Answer from the drawing. Dimensions are ordinates in mm from the lowest x, y and z of the part. A direction names the side the tool comes from. Round coordinates to 2 decimals unless told otherwise and drop trailing zeros. Loops run counter-clockwise (first coordinate to the right, second up) from the corner with the lowest first, then second, coordinate; pieces in that order, holes last.
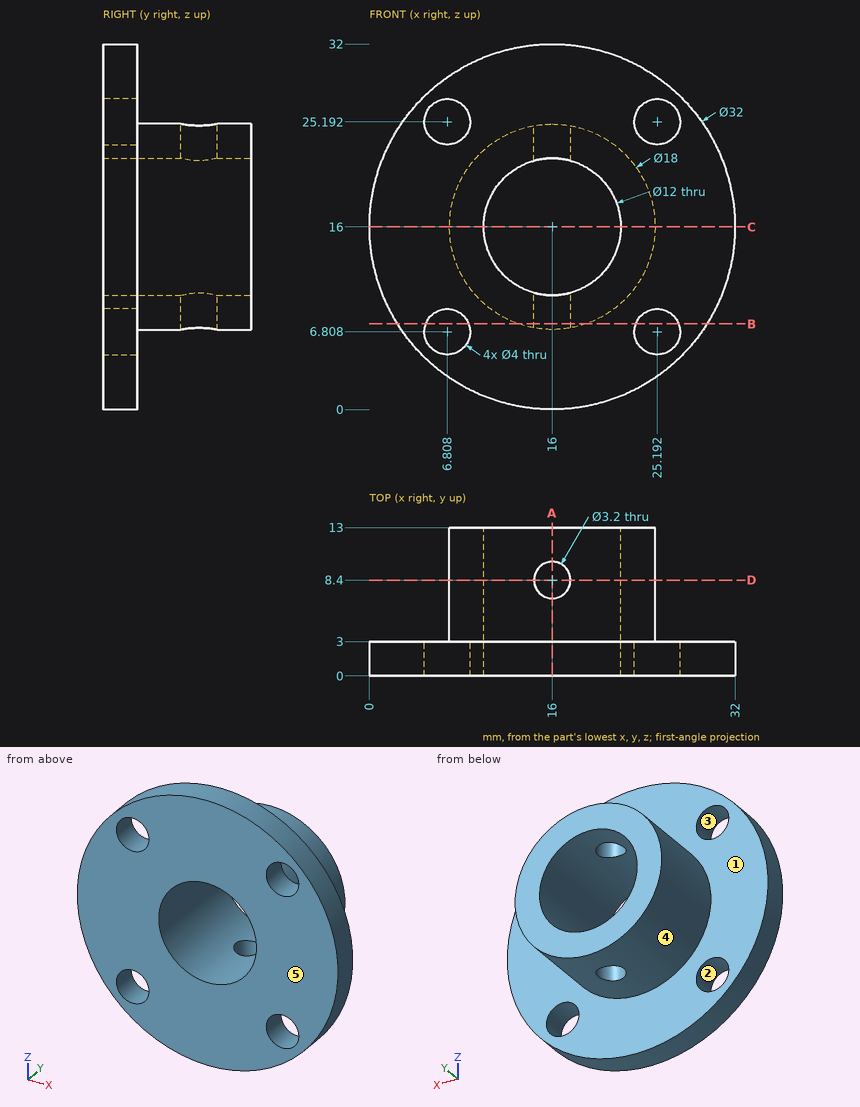
Item 1: Section A-A, the plane x = 16 is taken. Give the vertices of the cut face in (y, z), plus the area to 3 significant figures.
Item 2: Section D-D, the plane y = 8.4 is taken. Give the vertices of the cut face in (x, z), plus the area to 3 significant figures.
Item 3: Section B-B, the plane z = 7.5 is taken. Give the vertices of the cut face in (x, y) (1 decimal), plus the area to 3 significant figures.
Item 4: Determine the mould class of the marked faces 3, 4 and 5 for opening direction X: pulls with the +X half, pulls with the -X half, needs draft (parallel to the pull), parting line crosses it, or undercut.
Item 5: For the marked faces 1 and 2, determine the directions among +Z, -Z, +X, -X, +Y, -Y from which every point of the face is accessible in a straight line to the end or side of a thin tool.
Item 6: Section C-C, the plane z = 16 is taken. Give the vertices of the cut face in (x, y).
Item 7: Straight lines are drawn through the part: line 1 (Y direction, x = 30.5, z = 15); line 2 (Z direction, x = 20.5, y = 11.25) (1 decimal); line 3 (X direction, y = 8.4, z = 9.4). For each, find the intervals that lie inside material, in ascending order.
Item 8: Each of these flat-tipped pins is pushed along its axis until it touches: P1, Ø2, axis at y = 10, z = 9.5, coming from the -X side (1 decimal); P2, Ø1.5, axis at x = 24, y = 10, coming from the +Z side; P3, Ø6, axis at x = 9.5, y = 2.5, coming from the -Z side. Where does it stop, or does it pass through?
Answer below:
1. outline: (0, 0) - (3, 0) - (3, 7) - (6.8, 7) - (6.8, 10) - (0, 10) - close; (0, 22) - (6.8, 22) - (6.8, 25) - (3, 25) - (3, 32) - (0, 32) - close; (10, 7) - (13, 7) - (13, 10) - (10, 10) - close; (10, 22) - (13, 22) - (13, 25) - (10, 25) - close
1. area: 101 mm2
2. outline: (14.4, 7.14) - (14.4, 10.22) arc R6 cw to (14.4, 21.78) - (14.4, 24.86) arc R9 ccw to start; (17.6, 7.14) arc R9 ccw to (17.6, 24.86) - (17.6, 21.78) arc R6 cw to (17.6, 10.22) - close
2. area: 122 mm2
3. outline: (2.4, 0) - (4.9, 0) - (4.9, 3) - (2.4, 3) - close; (8.7, 0) - (23.3, 0) - (23.3, 3) - (19, 3) - (19, 13) - (13, 13) - (13, 3) - (8.7, 3) - close; (27.1, 0) - (29.6, 0) - (29.6, 3) - (27.1, 3) - close; hole circle Ø3.2 at (16, 8.4)
3. area: 110 mm2
4. face 3: undercut
4. face 4: parting line crosses it
4. face 5: needs draft
5. face 1: +Y
5. face 2: +Y, -Y
6. outline: (0, 0) - (10, 0) - (10, 13) - (7, 13) - (7, 3) - (0, 3) - close; (22, 0) - (32, 0) - (32, 3) - (25, 3) - (25, 13) - (22, 13) - close
7. line 1: y = 0 to 3
7. line 2: z = 8.2 to 12, 20 to 23.8
7. line 3: x = 9.88 to 14.4, 17.6 to 22.12
8. P1: stops at x = 8.9
8. P2: stops at z = 21.33
8. P3: stops at z = 0.39
